Design review of the part shown in the three views and the two pictorial views. Dimensions are in mm from the part's minimum x, y and z. A direction names the side the tool comes from. Round coordinates to 2 decimals unless told otherwise and drop trailing zeros. Write each loop counter-clockwise with the first axis right and the second up, starting at its lowest first coordinate (ties: lowest second). Pieces come first, ordered by that corner, then holes. Notation, with made-up numbers: (61, 42) - (71, 42) arc R23 cw to (71, 70) - close; hole circle Ø8 at (28, -37). An arc over 180 degrees is marked (long way). Use one line per item in the form item = value.
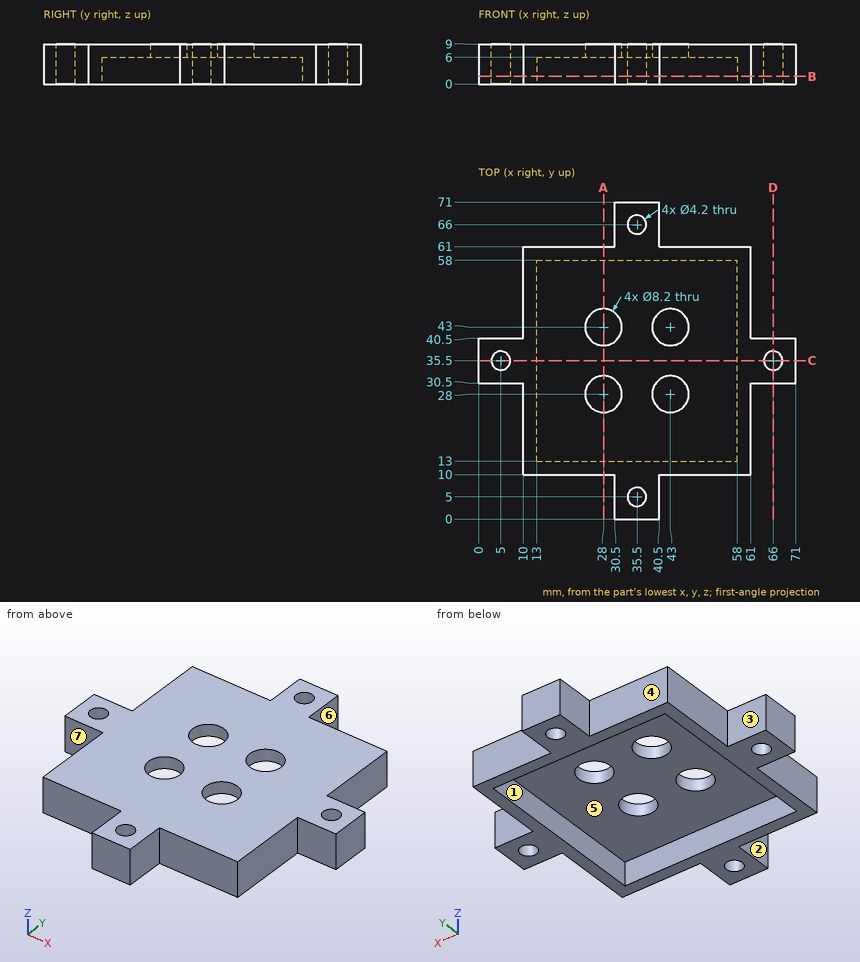
Q1. We need section D-D on x = 66. Write out the cut boundary in (y, z).
Calculated:
outline = (30.5, 0) - (33.4, 0) - (33.4, 9) - (30.5, 9) - close; (37.6, 0) - (40.5, 0) - (40.5, 9) - (37.6, 9) - close
Q2. To check wall thickness, follow line 1 along Y through (x, z) = (28, 7.25); line 2 along X through (y, z) = (66, 3); line 3 along Y through (x, z) = (53.5, 4.5). State the ranges of each line that lie inside material, in increasing order. Write a range as from..to.
Calculated:
line_1 = 10..23.9, 32.1..38.9, 47.1..61
line_2 = 30.5..33.4, 37.6..40.5
line_3 = 10..13, 58..61
Q3. We need section B-B on z = 1.75. Write out the cut boundary in (x, y), then the cut area to 3 significant figures.
Calculated:
outline = (0, 30.5) - (10, 30.5) - (10, 10) - (30.5, 10) - (30.5, 0) - (40.5, 0) - (40.5, 10) - (61, 10) - (61, 30.5) - (71, 30.5) - (71, 40.5) - (61, 40.5) - (61, 61) - (40.5, 61) - (40.5, 71) - (30.5, 71) - (30.5, 61) - (10, 61) - (10, 40.5) - (0, 40.5) - close; hole circle Ø4.2 at (5, 35.5); hole (13, 13) - (58, 13) - (58, 58) - (13, 58) - close; hole circle Ø4.2 at (35.5, 5); hole circle Ø4.2 at (35.5, 66); hole circle Ø4.2 at (66, 35.5)
area = 921 mm2
Q4. Machinability: for the marked faces 4, 5, 6 and 7, which of the approach directions +Z, -Z, +X, -X, +Y, -Y give a long, thin tool a straight path to every point of the face, cutting with its end or side? Answer none if there is none.
Calculated:
face_4 = +Z, -Z, -X, +Y
face_5 = -Z
face_6 = +Z, -Z, +X, +Y
face_7 = +Z, -Z, -X, -Y
Q5. Draft analysis for pull direction X (two halves, no side actions). For the marked faces 1, 2 and 3, state which applies: released by +X, released by -X, zero draft, split by the parting line, or undercut.
Calculated:
face_1 = undercut
face_2 = released by -X
face_3 = zero draft
Q6. We need section C-C on y = 35.5. Write out the cut boundary in (x, z).
Calculated:
outline = (0, 0) - (2.9, 0) - (2.9, 9) - (0, 9) - close; (7.1, 0) - (13, 0) - (13, 6) - (58, 6) - (58, 0) - (63.9, 0) - (63.9, 9) - (7.1, 9) - close; (68.1, 0) - (71, 0) - (71, 9) - (68.1, 9) - close
Q7. For P1, Ø7.5, axis at x = 43, y = 43, coming from the -Z side; P2, Ø4.5, axis at x = 67, z = 2.5, coming from the +Y side; P3, Ø1.8, axis at x = 37, z = 1.5, coming from the -Y side; P4, Ø2.5, axis at x = 51, z = 3.5, coming from the +Y side, all flat-tipped, find the tip position at first contact; note any pin that passes through.
Calculated:
P1 = through
P2 = 40.5
P3 = 0
P4 = 61
Q8. We need section A-A on x = 28. Write out the cut boundary in (y, z).
Calculated:
outline = (10, 0) - (13, 0) - (13, 6) - (23.9, 6) - (23.9, 9) - (10, 9) - close; (32.1, 6) - (38.9, 6) - (38.9, 9) - (32.1, 9) - close; (47.1, 6) - (58, 6) - (58, 0) - (61, 0) - (61, 9) - (47.1, 9) - close
